```python
from build123d import *

# Parameters (mm, degrees)
SKETCH2_R           = 4
BOSS_EXTRUDE2_DEPTH = 8


with BuildPart() as part:
    # Sketch2 → Boss-Extrude2 (new, symmetric)
    with BuildSketch(Plane(origin=(0, 0, 0), x_dir=(1, 0, 0), z_dir=(0, 1, 0))):
        with BuildLine():
            Line((-1.5, 15.929532322), (-1.5, 32.465366161))
            ThreePointArc((-1.5, 32.465366161), (-32.5, 0), (-1.5, -32.465366161))
            Line((-1.5, -32.465366161), (-1.5, -15.929532322))
            ThreePointArc((-1.5, -15.929532322), (-16, 0), (-1.5, 15.929532322))
        make_face()
        with Locations(Location((-24, 0, 0), (0, 0, 270))):
            Circle(SKETCH2_R, mode=Mode.SUBTRACT)
    extrude(amount=BOSS_EXTRUDE2_DEPTH, both=True)


solid = part.part
```
The listing builds one solid part. Answer for the finished solid, in the listing's coordinates (mm). Give positions to 0.01 mm unless a question says otherwise; leave off trailing zeros. Order: outer loops, then holes, each group sorted by start corner. A loop starts at its lowest first (then second) coordinate and runs counter-clockwise, first axis right, second up.
Item 1: Given pin 1 Ø3 at (x, y) = (-15.5, -4) entering from -Z; pin 2 Ø1.5 at (x, y) = (-29, -2.5) entering from +Z; pin 3 Ø2 at (x, y) = (-8.5, 1) entering from -Z, each flat-ended and moving along its own axis, determine where each tip first touches the part or whether it passes through.
From the geometry:
pin 1: stops at z = -29.33
pin 2: stops at z = 16.07
pin 3: stops at z = -31.62
Item 2: For a pull along Z with two mould halves and no side action, classify faces 1 (the face through (-17, 8, 0)), 2 (the face through (-32.493, 0.112, -0.694)), 3 (the face through (-16, 0, 0)) as pulls with the +Z half, pulls with the -Z half, needs draft (parallel to the pull), parting line crosses it, or undercut.
From the geometry:
face 1: needs draft
face 2: parting line crosses it
face 3: undercut
Item 3: The part is cut by section D-D, the plane x = -30. Give the vertices of the cut face in (y, z).
From the geometry:
outline: (-8, -12.5) - (8, -12.5) - (8, 12.5) - (-8, 12.5) - close
Item 4: The part is cut by section B-B, the plane x = -24. Give the vertices of the cut face in (y, z).
From the geometry:
outline: (-8, -21.91) - (8, -21.91) - (8, -4) - (-8, -4) - close; (-8, 4) - (8, 4) - (8, 21.91) - (-8, 21.91) - close
Item 5: Find the intervals of material crossed by probe 1 along Z at (x, y) = (-21, -2.5); probe 2 along Z at (x, y) = (-10, 0.25); probe 3 along X at (y, z) = (-6, -0.5), in increasing order.
From the geometry:
probe 1: z = -24.8 to -2.65, 2.65 to 24.8
probe 2: z = -30.92 to -12.49, 12.49 to 30.92
probe 3: x = -32.5 to -27.97, -20.03 to -15.99
Item 6: The part is cut by section A-A, the plane z = 0. Give the vertices of the cut face in (x, y).
From the geometry:
outline: (-32.5, -8) - (-28, -8) - (-28, 8) - (-32.5, 8) - close; (-20, -8) - (-16, -8) - (-16, 8) - (-20, 8) - close
